```python
from build123d import *

# Parameters (mm, degrees)
F3_DEPTH = 6
F4_R     = 1


with BuildPart() as f1:
    # F0 (on Front) → F1 (revolve)
    with BuildSketch(Plane.XZ):
        with BuildLine():
            Line((-14.5940445242, 0), (0, 0))
            Line((0, 0), (0, 6))
            Line((0, 6), (-2, 6))
            Line((-2, 6), (-2, 3))
            Line((-2, 3), (-11, 3))
            Line((-11, 3), (-12.6100640914, 3.1408623555))
            ThreePointArc((-12.6100640914, 3.1408623555), (-13.7813661664, 2.8822577685), (-14.5940445242, 2))
            Line((-14.5940445242, 2), (-14.5940445242, 0))
        make_face()
    revolve(axis=Axis((-7.2970222621, 0, 0), (1, 0, 0)))

    # F2 (on face) → F3 (cut)
    with BuildSketch(Plane(origin=(-14.5940445242, 0, 0), x_dir=(0, -1, 0), z_dir=(-1, 0, 0))):
        with BuildLine():
            ThreePointArc((-1.9691368668, -0.35), (-2, 0), (-1.9691368668, 0.35))
            Line((-1.9691368668, 0.35), (-4, 0.35))
            Line((-4, 0.35), (-4, -0.35))
            Line((-4, -0.35), (-2.9795133831, -0.35))
            Line((-2.9795133831, -0.35), (-1.9691368668, -0.35))
        make_face()
        with BuildLine():
            Line((1.9691368668, 0.35), (0.25, 0.35))
            Line((0.25, 0.35), (0.25, 0))
            Line((0.25, 0), (0.25, -0.35))
            Line((0.25, -0.35), (1.9691368668, -0.35))
            ThreePointArc((1.9691368668, -0.35), (1.9922692757, -0.1756790632), (2, 0))
            ThreePointArc((2, 0), (1.9922692757, 0.1756790632), (1.9691368668, 0.35))
        make_face()
        with BuildLine():
            Line((-0.25, 0), (-0.25, 0.35))
            Line((-0.25, 0.35), (-1.9691368668, 0.35))
            ThreePointArc((-1.9691368668, 0.35), (-2, 0), (-1.9691368668, -0.35))
            Line((-1.9691368668, -0.35), (-0.25, -0.35))
            Line((-0.25, -0.35), (-0.25, 0))
        make_face()
        Polygon((0.25, 0), (0.25, 0.35), (-0.25, 0.35), (-0.25, 0), (-0.25, -0.35), (0.25, -0.35), align=None)
        with BuildLine():
            Line((4, 0.35), (1.9691368668, 0.35))
            ThreePointArc((1.9691368668, 0.35), (1.9922692757, 0.1756790632), (2, 0))
            ThreePointArc((2, 0), (1.9922692757, -0.1756790632), (1.9691368668, -0.35))
            Line((1.9691368668, -0.35), (2.9795133831, -0.35))
            Line((2.9795133831, -0.35), (4, -0.35))
            Line((4, -0.35), (4, 0.35))
        make_face()
    extrude(amount=-F3_DEPTH, mode=Mode.SUBTRACT)

    # F4
    f4_edges = [f1.edges().sort_by_distance(p)[0] for p in [
        (-2, 0, -3),
    ]]
    fillet(f4_edges, radius=F4_R)


solid = f1.part
```
Geometry: final body of the model. Coordinates: model frame, mm. A direction names the side the tool comes from. Round coordinates to 2 decimals unless told otherwise and drop trailing zeros. Order: outer loops, then holes, each group sorted by start corner. A loop starts at its lowest first (then second) coordinate and runs counter-clockwise, first axis right, second up. Notation, with made-up numbers: (22.25, -23) -> (41.25, -23) arc R16 ccw to (41.25, -19) -> close; hole circle Ø8 at (49.5, -31). An arc over 180 degrees is marked (long way). Use one line per item in the form item = value.
(1) Access query for faces 1 (the face through (-2, 3.92, -1.42)), 2 (the face through (-11.82, 0.06, 3.07)), 3 (the face through (-12, 0, 0.35)), 4 (the face through (-11.82, -0.06, -3.07)), 5 (the face through (-7, 0, -3)). Directions: +Z, -Z, +X, -X, +Y, -Y. A direction counts if a zero-diameter tool reaches every point of the face in a straight line with its end or side. Return the directions, or none.
Results list:
face_1 = -X
face_2 = +Z
face_3 = -X, +Y, -Y
face_4 = -Z
face_5 = none
(2) Draft query along Z for faces 6 (the face through (-1, 0, -6)), 7 (the face through (-14.594, 0, -1)), 8 (the face through (-12, 0, -0.35)). Return one class per face: pulls with the +Z half, pulls with the -Z half, needs draft (parallel to the pull), parting line crosses it, or undercut.
Results list:
face_6 = parting line crosses it
face_7 = needs draft
face_8 = undercut
(3) First-contact query: pin 1 Ø1.5 at (x, z) = (-3.5, 2) entering from -Y; pin 2 Ø6 at (y, z) = (2.5, -3.5) entering from +X; pin 3 Ø5 at (x, z) = (-2, -4.5) entering from -Y; pin 4 Ø6 at (x, y) = (-9.5, -4.5) entering from +Z. Flat tips, straight axial feed; report the tip coordinate or a pass-through.
Results list:
pin_1 = -2.73
pin_2 = 0
pin_3 = -5.66
pin_4 = 2.6
(4) Section A-A on z = 0. Return loops of the section in (x, y), and give its area (3 significant figures).
Results list:
outline = (-8.59, -3) -> (-3, -3) arc R1 cw to (-2, -4) -> (-2, -6) -> (0, -6) -> (0, 6) -> (-2, 6) -> (-2, 4) arc R1 cw to (-3, 3) -> (-8.59, 3) -> close
area = 64.0 mm^2
(5) Section C-C on x = -5. Return loops of the section in (y, z).
Results list:
outline = circle Ø6 at (0, 0)
(6) Ray query, probe 1 along X at (y, z) = (3.25, -3.75); probe 2 along Z at (x, y) = (-6.5, 0); probe 3 along Z at (x, y) = (-11.5, 0.25). Return the intervals inside material, ascending. Write a range as [from, to].
Results list:
probe_1 = [-2, 0]
probe_2 = [-3, 3]
probe_3 = [-3.03, -0.35], [0.35, 3.03]
(7) Section B-B on x = -11.5. Return loops of the section in (y, z), and give its area (3 significant figures).
Results list:
outline = (-3.02, -0.35) arc R3.04 ccw to (3.02, -0.35) -> close; (-3.02, 0.35) -> (3.02, 0.35) arc R3.04 ccw to start
area = 24.9 mm^2
